CAD build for the part. Positions are in the model's coordinates, mm. Round coordinates to 2 decimals unless told otherwise and drop trailing zeros. Loops run counter-clockwise (first coordinate to the right, second up) from the corner with the lowest first, then second, coordinate; pieces in that order, holes last. Notation, with made-up numbers: M -5,-11 L 28,-11 A19 ccw 28,13 Z; hole C -12,48.25 d6. An arc over 180 degrees is marked long. One line per item, written item: value. Start each with the question number.
from build123d import *

# Parameters (mm, degrees)
SKETCH_1_R          = 3.6
EXTRUDE_1_DEPTH     = 15.5
SKETCH_2_R          = 5
CUT_EXTRUDE_1_DEPTH = 31.5


with BuildPart() as part:
    # 草图1 → 凸台-拉伸1 (new body)
    with BuildSketch(Plane(origin=(0, 0, 0), x_dir=(1, 0, 0), z_dir=(0, 1, 0))):
        with BuildLine():
            Line((27.835232693, 2.164767307), (10.503072433, 14.617984453))
            ThreePointArc((10.503072433, 14.617984453), (0, 18), (-10.503072433, 14.617984453))
            Line((-10.503072433, 14.617984453), (-27.835232693, 2.164767307))
            ThreePointArc((-27.835232693, 2.164767307), (-30, 0), (-27.835232693, -2.164767307))
            Line((-27.835232693, -2.164767307), (-10.503072433, -14.617984453))
            ThreePointArc((-10.503072433, -14.617984453), (0, -18), (10.503072433, -14.617984453))
            Line((10.503072433, -14.617984453), (27.835232693, -2.164767307))
            ThreePointArc((27.835232693, -2.164767307), (30, 0), (27.835232693, 2.164767307))
        make_face()
        with Locations(Location((-22.5, 0, 0), (0, 0, 270))):
            Circle(SKETCH_1_R, mode=Mode.SUBTRACT)
        with Locations(Location((22.5, 0, 0), (0, 0, 270))):
            Circle(SKETCH_1_R, mode=Mode.SUBTRACT)
    extrude(amount=EXTRUDE_1_DEPTH)

    # 草图2 → 切除-拉伸1 (cut)
    with BuildSketch(Plane(origin=(0, 15.5, 0), x_dir=(1, 0, 0), z_dir=(0, 1, 0))):
        with Locations(Location((0, 0, 0), (0, 0, 270))):
            Circle(SKETCH_2_R)
    extrude(amount=-CUT_EXTRUDE_1_DEPTH, mode=Mode.SUBTRACT)


solid = part.part
(1) Slice it at D-D, the plane x = 22.5. List the corners of the cut face in (y, z).
(2) Probe L1, parallel to X at y = 4, z = 0; L2, parallel to X at y = 11.5, z = 1; L3, parallel to X at y = 12.75, z = -9. List the from-to ranges inside material, lowest first.
(3) Slice it at A-A, the plane x = 0. List the corners of the cut face in (y, z), and give its area (3 significant figures).
(4) Mould opens along X. For faces 1 (the flat face through (-19.29, 7.642, 8.304)), 2 (the cylindrical face through (18.986, 7.642, -0.78)), 3 (the cylindrical face through (-4.88, 7.86, -1.08)), 4 (the cylindrical face through (0, 8, -18)) say: pulls with the +X half, pulls with the -X half, needs draft (parallel to the pull), parting line crosses it, or undercut.
(5) Flat gauge pins, fed straight in: P1, Ø8, axis at x = -8.5, y = 13, coming from the -Z side; P2, Ø2, axis at x = 18, y = 9, coming from the +Z side; P3, Ø6, axis at x = 22.5, z = 0, coming from the -Y side; P4, Ø1.5, axis at y = 6.5, z = -10.5, coming from the +X side. Where does each tip first touch, or does it go through?
(6) Slice it at B-B, the plane z = 0. List the corners of the cut face in (x, y).
(7) Slice it at C-C, the plane y = 12.75. List the corners of the cut face in (x, z), and give its area (3 significant figures).
Check result:
1. outline: M 0,-6 L 15.5,-6 L 15.5,-3.6 L 0,-3.6 Z; M 0,3.6 L 15.5,3.6 L 15.5,6 L 0,6 Z
2. L1: x = -30 to -26.1, -18.9 to -5, 5 to 18.9, 26.1 to 30
2. L2: x = -29.76 to -25.96, -19.04 to -4.9, 4.9 to 19.04, 25.96 to 29.76
2. L3: x = -18.32 to 18.32
3. outline: M 0,-18 L 15.5,-18 L 15.5,-5 L 0,-5 Z; M 0,5 L 15.5,5 L 15.5,18 L 0,18 Z
3. area: 403 mm^2
4. face 1: pulls with the -X half
4. face 2: undercut
4. face 3: undercut
4. face 4: parting line crosses it
5. P1: stops at z = -17.43
5. P2: stops at z = 9.95
5. P3: passes through
5. P4: stops at x = 17.28
6. outline: M -30,0 L -26.1,0 L -26.1,15.5 L -30,15.5 Z; M -18.9,0 L -5,0 L -5,15.5 L -18.9,15.5 Z; M 5,0 L 18.9,0 L 18.9,15.5 L 5,15.5 Z; M 26.1,0 L 30,0 L 30,15.5 L 26.1,15.5 Z
7. outline: M -27.84,-2.16 L -10.5,-14.62 A18 ccw 10.5,-14.62 L 27.84,-2.16 A2.16 ccw 27.84,2.16 L 10.5,14.62 A18 ccw -10.5,14.62 L -27.84,2.16 A2.16 ccw Z; hole C -22.5,0 d7.2; hole C 0,0 d10; hole C 22.5,0 d7.2
7. area: 1,150 mm^2
